Check sheet for the modelled part. Datum: model origin and axes. Units: mm. Coordinates: 2 decimals unless noted, no trailing zeros. Order: outer loops, then holes, each group sorted by start corner. A loop starts at its lowest first (then second) coordinate and runs counter-clockwise, first axis right, second up.
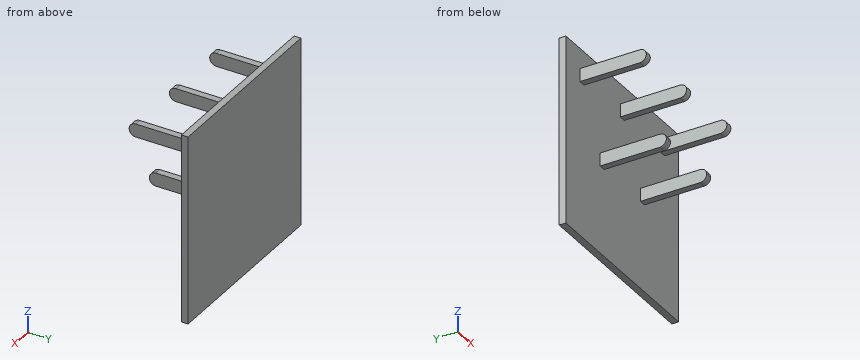
Autodesk Inventor part; units mm, degrees
ref_plane "pole_to_body_XY" through (0, 0.508, 0) normal (0, 1, 0) x (1, 0, 0)
ref_plane "pole_to_body_YZ" through (0, 0.508, 0) normal (1, 0, 0) x (0, 0, -1)
ref_plane "pole_to_body_ZX" through (0, 0.508, 0) normal (0, 0, -1) x (0, 1, 0)
sketch "Sketch_1" plane through (0, 0, 0) normal (0, 1, 0) x (-1, 0, 0)
  line L0 (7.112, -7.112) -> (7.112, 7.112)
  line L1 (7.112, 7.112) -> (-7.112, 7.112)
  line L2 (-7.112, 7.112) -> (-7.112, -7.112)
  line L3 (-7.112, -7.112) -> (7.112, -7.112)
extrude "Extrusion1" add sketch "Sketch_1" along normal blind 0.508
sketch "Sketch_10" plane through (-5.08, 0, 0) normal (1, 0, 0) x (0, 0, -1)
  arc A0 (-5.5753, -4.5085) -> (-5.08, -5.0038) centre (-5.08, -4.5085) ccw
  arc A1 (-5.08, -5.0038) -> (-4.5847, -4.5085) centre (-5.08, -4.5085) ccw
  line L0 (-4.5847, -4.5085) -> (-4.5847, 0.508)
  line L1 (-4.5847, 0.508) -> (-5.5753, 0.508)
  line L2 (-5.5753, 0.508) -> (-5.5753, -4.5085)
extrude "Extrusion2" add sketch "Sketch_10" along normal mid plane 0.508
sketch "Sketch_12" plane through (0, 0, 0) normal (1, 0, 0) x (0, 1, 0)
  arc A0 (-4.5085, 5.5753) -> (-5.0038, 5.08) centre (-4.5085, 5.08) ccw
  arc A1 (-5.0038, 5.08) -> (-4.5085, 4.5847) centre (-4.5085, 5.08) ccw
  line L0 (-4.5085, 4.5847) -> (0.508, 4.5847)
  line L1 (0.508, 4.5847) -> (0.508, 5.5753)
  line L2 (0.508, 5.5753) -> (-4.5085, 5.5753)
extrude "Extrusion3" add sketch "Sketch_12" along normal mid plane 0.508
sketch "Sketch_14" plane through (5.08, 0, 0) normal (1, 0, 0) x (0, 0, -1)
  arc A0 (-5.5753, -4.5085) -> (-5.08, -5.0038) centre (-5.08, -4.5085) ccw
  arc A1 (-5.08, -5.0038) -> (-4.5847, -4.5085) centre (-5.08, -4.5085) ccw
  line L0 (-4.5847, -4.5085) -> (-4.5847, 0.508)
  line L1 (-4.5847, 0.508) -> (-5.5753, 0.508)
  line L2 (-5.5753, 0.508) -> (-5.5753, -4.5085)
extrude "Extrusion4" add sketch "Sketch_14" along normal mid plane 0.508
sketch "Sketch_16" plane through (-2.54, 0, 0) normal (1, 0, 0) x (0, 0, -1)
  line L0 (-0.4953, 0.508) -> (-0.4953, -4.5085)
  arc A0 (-0.4953, -4.5085) -> (0, -5.0038) centre (0, -4.5085) ccw
  arc A1 (0, -5.0038) -> (0.4953, -4.5085) centre (0, -4.5085) ccw
  line L1 (0.4953, -4.5085) -> (0.4953, 0.508)
  line L2 (0.4953, 0.508) -> (-0.4953, 0.508)
extrude "Extrusion5" add sketch "Sketch_16" along normal mid plane 0.508
sketch "Sketch_17" plane through (2.54, 0, 0) normal (1, 0, 0) x (0, 0, -1)
  line L0 (-0.4953, 0.508) -> (-0.4953, -4.5085)
  arc A0 (-0.4953, -4.5085) -> (0, -5.0038) centre (0, -4.5085) ccw
  arc A1 (0, -5.0038) -> (0.4953, -4.5085) centre (0, -4.5085) ccw
  line L1 (0.4953, -4.5085) -> (0.4953, 0.508)
  line L2 (0.4953, 0.508) -> (-0.4953, 0.508)
extrude "Extrusion6" add sketch "Sketch_17" along normal mid plane 0.508
ref_plane "pole_to_body_XY" through (0, 0.508, 0) normal (0, 1, 0) x (1, 0, 0)
ref_plane "pole_to_body_YZ" through (0, 0.508, 0) normal (1, 0, 0) x (0, 0, -1)
ref_plane "pole_to_body_ZX" through (0, 0.508, 0) normal (0, 0, -1) x (0, 1, 0)
properties part number "UB21G035D-1JBpole"
(1) Cross-section at B-B (x = 5). Enter the section's corners in (y, z), and give its area (3 significant figures).
Filled in:
outline: (-4.51, 4.58) - (0, 4.58) - (0, -7.11) - (0.51, -7.11) - (0.51, 7.11) - (0, 7.11) - (0, 5.58) - (-4.51, 5.58) arc R0.5 ccw to start
area: 12.1 mm2
(2) Go/stop test with flat-tipped pins: P1, Ø0.6, axis at x = -2.5, y = -1.5, coming from the +Z side; P2, Ø0.6, axis at x = 2.5, y = -3.5, coming from the -Z side; P3, Ø0.5, axis at y = -3.5, z = 0, coming from the +X side. Record where each tip stops, or that it passes through.
Filled in:
P1: stops at z = 0.5
P2: stops at z = -0.5
P3: stops at x = 2.79
(3) Cross-section at D-D (x = -3). Enter the section's corners in (y, z).
Filled in:
outline: (0, -7.11) - (0.51, -7.11) - (0.51, 7.11) - (0, 7.11) - close
(4) Cross-section at C-C (z = 5.08). Enter the section's corners in (x, y).
Filled in:
outline: (-7.11, 0) - (-5.33, 0) - (-5.33, -5) - (-4.83, -5) - (-4.83, 0) - (-0.25, 0) - (-0.25, -5) - (0.25, -5) - (0.25, 0) - (4.83, 0) - (4.83, -5) - (5.33, -5) - (5.33, 0) - (7.11, 0) - (7.11, 0.51) - (-7.11, 0.51) - close
(5) Thickness scan on probe 1 along X at (y, z) = (-1.8, 5); probe 2 along Y at (x, z) = (-3.5, 4.5); probe 3 along Z at (x, y) = (-5.25, -1.4). Record the ranges inside material, lowest first.
Filled in:
probe 1: x = -5.33 to -4.83, -0.25 to 0.25, 4.83 to 5.33
probe 2: y = 0 to 0.51
probe 3: z = 4.58 to 5.58
(6) Cross-section at A-A (y = -3.2). Enter the section's corners in (x, z), and give its area (3 significant figures).
Filled in:
outline: (-5.33, 4.58) - (-4.83, 4.58) - (-4.83, 5.58) - (-5.33, 5.58) - close; (-2.79, -0.5) - (-2.29, -0.5) - (-2.29, 0.5) - (-2.79, 0.5) - close; (-0.25, 4.58) - (0.25, 4.58) - (0.25, 5.58) - (-0.25, 5.58) - close; (2.29, -0.5) - (2.79, -0.5) - (2.79, 0.5) - (2.29, 0.5) - close; (4.83, 4.58) - (5.33, 4.58) - (5.33, 5.58) - (4.83, 5.58) - close
area: 2.52 mm2
